from build123d import *

# Parameters (mm, degrees)
SKETCH_1_R          = 6
EXTRUDE_1_DEPTH     = 5
SKETCH_2_W          = 3
SKETCH_2_H          = 15
EXTRUDE_2_DEPTH     = 90
SKETCH_4_R          = 4
CUT_EXTRUDE_1_DEPTH = 46.5
SKETCH_5_R          = 10
SKETCH_5_R_2        = 6
EXTRUDE_3_DEPTH     = 10


with BuildPart() as part:
    # 草圖1 → 填料-伸長1 (new body)
    with BuildSketch(Plane.XY):
        Polygon((-22.5, -2.5), (-22.5, -10), (22.5, -10), (22.5, -2.5), (27.5, -2.5), (27.5, 2.5), (22.5, 2.5), (22.5, 10), (-22.5, 10), (-22.5, 2.5), (-27.5, 2.5), (-27.5, -2.5), align=None)
        Circle(SKETCH_1_R, mode=Mode.SUBTRACT)
    extrude(amount=EXTRUDE_1_DEPTH)

    # 草圖2 → 填料-伸長2 (add)
    with BuildSketch(Plane(origin=(0, 0, 0), x_dir=(-1, 0, 0), z_dir=(0, 0, -1))):
        with Locations((-16.5, 0)):
            Rectangle(SKETCH_2_W, SKETCH_2_H)
        with Locations((16.5, 0)):
            Rectangle(SKETCH_2_W, SKETCH_2_H)
    extrude(amount=EXTRUDE_2_DEPTH)

    # 草圖4 → 除料-伸長1 (cut, through all)
    with BuildSketch(Plane(origin=(18, 0, 0), x_dir=(0, 0, -1), z_dir=(1, 0, 0))):
        with Locations((82.5, 0)):
            Circle(SKETCH_4_R)
    extrude(amount=-CUT_EXTRUDE_1_DEPTH, mode=Mode.SUBTRACT)

    # 草圖5 → 填料-伸長3 (add)
    with BuildSketch(Plane(origin=(0, 0, 0), x_dir=(-1, 0, 0), z_dir=(0, 0, -1))):
        Circle(SKETCH_5_R)
        Circle(SKETCH_5_R_2, mode=Mode.SUBTRACT)
    extrude(amount=EXTRUDE_3_DEPTH)


solid = part.part
Build history of the part. All positions in model axes, mm. A direction names the side the tool comes from. Coordinates: 2 decimals unless noted, no trailing zeros. Write each loop counter-clockwise with the first axis right and the second up, starting at its lowest first coordinate (ties: lowest second). Pieces come first, ordered by that corner, then holes. Notation, with made-up numbers: (72.5, 51.25) -> (94.5, 51.25) arc R12 cw to (94.5, 55.25) -> close; hole circle Ø4 at (81, 38.25). An arc over 180 degrees is marked (long way). Use CSV: the item, a comma, the result in double quotes. Start each with the question number.
Q1. Cut at D-D, the plane x = -5. List the corners of the cut face in (y, z).
Q2. Cut at C-C, the plane z = -70. List the corners of the cut face in (x, y), then the cut area to 3 significant figures.
Q3. Cut at B-B, the plane z = -82.5. List the corners of the cut face in (x, y).
Q4. Cut at A-A, the plane z = -6.5. List the corners of the cut face in (x, y).
Q5. 3-axis set-ups, long thin cutter, end or side, ignore diameter. For faces 1 (the cylindrical face through (-16.479, 0.176, -78.504)), 2 (the flat face through (25, 2.5, 2)), 3 (the flat face through (-22.5, -6, 2)), 4 (the flat face through (-18, 0, -44)), 5 (the flat face through (-22.5, 6, 2)): which of +Z, -Z, +X, -X, +Y, -Y reach the whole face in a straight line?
Q6. Drill centre lines: probe 1 along X at (y, z) = (0, -6.5); probe 2 along X at (y, z) = (-2.5, -47.5); probe 3 along X at (y, z) = (0, 1). Where is each one in solid material? Low to high.
Q7. Pull direction X, two halves, no side cores. Call faces 6 (the flat face through (-27.5, 0, 2)), 7 (the flat face through (-15, 0, -44)), 8 (the flat face through (-16, -7.5, -44)): released by +X, released by -X, zero draft, split by the parting line, or undercut.
Q8. Flat gauge pins, fed straight in: pin 1 Ø10 at (y, z) = (-6.5, -24.5) entering from +X; pin 2 Ø6 at (x, z) = (20, -57.5) entering from -Y; pin 3 Ø5.5 at (y, z) = (6, 2) entering from +X; pin 4 Ø6.5 at (y, z) = (0, -82.5) entering from +X. Where does each tip first touch, or does it go through?
Checked values:
1,outline,"(-10, 0) -> (-8.66, 0) -> (-8.66, -10) -> (-3.32, -10) -> (-3.32, 5) -> (-10, 5) -> close; (3.32, -10) -> (8.66, -10) -> (8.66, 0) -> (10, 0) -> (10, 5) -> (3.32, 5) -> close"
2,outline,"(-18, -7.5) -> (-15, -7.5) -> (-15, 7.5) -> (-18, 7.5) -> close; (15, -7.5) -> (18, -7.5) -> (18, 7.5) -> (15, 7.5) -> close"
2,area,"90.0 mm²"
3,outline,"(-18, -7.5) -> (-15, -7.5) -> (-15, -4) -> (-18, -4) -> close; (-18, 4) -> (-15, 4) -> (-15, 7.5) -> (-18, 7.5) -> close; (15, -7.5) -> (18, -7.5) -> (18, -4) -> (15, -4) -> close; (15, 4) -> (18, 4) -> (18, 7.5) -> (15, 7.5) -> close"
4,outline,"(-18, -7.5) -> (-15, -7.5) -> (-15, 7.5) -> (-18, 7.5) -> close; circle Ø20 at (0, 0); (15, -7.5) -> (18, -7.5) -> (18, 7.5) -> (15, 7.5) -> close; hole circle Ø12 at (0, 0)"
5,face 1,"+X, -X"
5,face 2,"+Z, -Z, +X, +Y"
5,face 3,"+Z, -Z, -X, -Y"
5,face 4,"-Z, -X, +Y, -Y"
5,face 5,"+Z, -Z, -X, +Y"
6,probe 1,"x = -18 to -15, -10 to -6, 6 to 10, 15 to 18"
6,probe 2,"x = -18 to -15, 15 to 18"
6,probe 3,"x = -27.5 to -6, 6 to 27.5"
7,face 6,"released by -X"
7,face 7,"undercut"
7,face 8,"zero draft"
8,pin 1,"stops at x = 18"
8,pin 2,"stops at y = -7.5"
8,pin 3,"stops at x = 22.5"
8,pin 4,"passes through"
